```python
from build123d import *


with BuildPart() as part:
    # Esquisse1 → Révolution1 (revolve)
    with BuildSketch(Plane.XY, mode=Mode.PRIVATE) as r_volution1_sk:
        Polygon((2.777777778, -1.6), (3.5, -1.6), (3.5, -1.2), (3, -1.2), (2, -0.3), (1.4, -0.3), (1.4, 0.3), (2, 0.3), (3, 1.2), (3.5, 1.2), (3.5, 1.6), (2.777777778, 1.6), (2, 0.9), (1, 0.9), (1, -2.4), (1.4, -2.4), (1.4, -0.9), (2, -0.9), align=None)
    revolve(r_volution1_sk.sketch.rotate(Axis((0, 0, 0), (0, 1, 0)), 90), axis=Axis((0, 0, 0), (0, 1, 0)))


solid = part.part
```
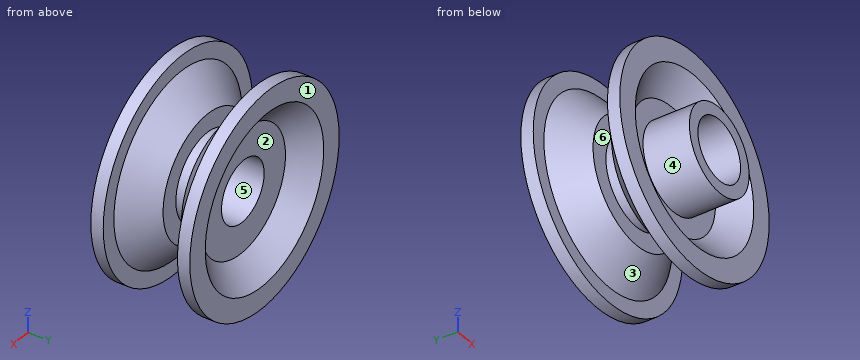
Build history of the part. All positions in model axes, mm. Face numbers are marked on the shaded views. A direction names the side the tool comes from. Give positions to 0.01 mm unless a question says otherwise; leave off trailing zeros. One line per question, with ' | ' between items. Start each with the question number.
1) Pin check, flat tips, straight feed: pin 1 (3 mm diameter, centred on x = 0.5, z = 1, fed in from +Y); pin 2 (2 mm diameter, centred on x = 1, z = 0.5, fed in from +Y). Stop position of each tip, or through.
2) Two-plate mould, pull along Z, no slides. Class the marked faces 1, 2 and 3: released by +Z, released by -Z, zero draft, split by the parting line, or undercut.
3) 3-axis set-ups, long thin cutter, end or side, ignore diameter. For the marked faces 4, 5 and 6: which of +Z, -Z, +X, -X, +Y, -Y reach the whole face in a straight line?
4) Probe L1, parallel to X at y = -1.7, z = 0; L2, parallel to Z at x = -0.5, y = -1.05; L3, parallel to Y at x = 0.5, z = -1.75. List the from-to ranges inside material, lowest first.
Return value:
1) pin 1: y = 1.46 | pin 2: y = 1.01
2) face 1: zero draft | face 2: undercut | face 3: split by the parting line
3) face 4: -Y | face 5: +Y, -Y | face 6: none
4) L1: -1.4 to -1, 1 to 1.4 | L2: -2.79 to -2.11, -1.31 to -0.87, 0.87 to 1.31, 2.11 to 2.79 | L3: -0.9 to -0.3, 0.3 to 0.9
